Could you check a few things on this model? Use its own coordinates, in mm. Face numbers are marked on the shaded views. Round coordinates to 2 decimals unless told otherwise and drop trailing zeros. Order: outer loops, then holes, each group sorted by start corner. A loop starts at its lowest first (then second) coordinate and runs counter-clockwise, first axis right, second up. Notation, with made-up numbers: (89, 4) - (123, 4) arc R23 cw to (123, 43) - close; hole circle Ø5 at (-28.5, 75.5). An arc over 180 degrees is marked (long way). Use one line per item in the form item = value.
from build123d import *

# Parameters (mm, degrees)
EXTRUDE1_DEPTH          = 6.35
EXTRUDE1_DEPTH_BACK     = 6.35
SKETCH1_R               = 1.4224
SKETCH8_OUTSIDE_W       = 58.916
SKETCH8_OUTSIDE_H       = 59.654
SKETCH8_OUTSIDE_R       = 2.38125
EXTRUDE4_DEPTH          = 14.210632851
EXTRUDE4_DRAFT          = -60
MIRROR1_COPY_1_SKETCH_W = 58.916
MIRROR1_COPY_1_SKETCH_H = 59.654
MIRROR1_COPY_1_SKETCH_R = 2.38125
MIRROR1_COPY_1_DEPTH    = 14.210632851
MIRROR1_COPY_1_DRAFT    = -60


with BuildPart() as part:
    # Sketch1 → Extrude1 (new, two sides: drawn at the far end of the back side and taken through both)
    with BuildSketch(Plane.XY.offset(-EXTRUDE1_DEPTH_BACK)):
        Polygon((0, 2.749630657), (-2.38125, 1.374815329), (-2.38125, -1.374815329), (0, -2.749630657), (2.38125, -1.374815329), (2.38125, 1.374815329), align=None)
        Circle(SKETCH1_R, mode=Mode.SUBTRACT)
    extrude(amount=EXTRUDE1_DEPTH + EXTRUDE1_DEPTH_BACK)

    # Extrude3 cone 1 section (through the dimple's axis) → Extrude3 (revolve, cut)
    with BuildSketch(Plane(origin=(0, 0, -6.35), x_dir=(0, 1, 0), z_dir=(1, 0, 0))):
        Polygon((0, 0), (1.4732, 0), (0, 1.579813584), align=None)
    extrude3 = revolve(axis=Axis((0, 0, -6.35), (0, 0, 1)), mode=Mode.SUBTRACT)


with BuildPart() as extrude4_tool:
    # Sketch8 outside → Extrude4 (with draft: the straight prism first)
    with BuildSketch(Plane(origin=(0, 0, -6.35), x_dir=(-1, 0, 0), z_dir=(0, 0, -1))):
        Rectangle(SKETCH8_OUTSIDE_W, SKETCH8_OUTSIDE_H)
        Circle(SKETCH8_OUTSIDE_R, mode=Mode.SUBTRACT)
    extrude(amount=-EXTRUDE4_DEPTH)
    # Extrude4: the draft: its side faces are tilted about the plane it starts from
    extrude4_sides = [extrude4_tool.faces().sort_by_distance(p)[0] for p in [
        (0, -29.827, 0.755316425),
        (-29.458, 0, 0.755316425),
        (0, 29.827, 0.755316425),
        (29.458, 0, 0.755316425),
        (2.38125, 0, 0.755316425),
    ]]
    draft(extrude4_sides, Plane(origin=(0, 0, -6.35), x_dir=(-1, 0, 0), z_dir=(0, 0, -1)), EXTRUDE4_DRAFT)


with BuildPart() as part_1:
    add(part.part)

    # Extrude4: cut by extrude4_tool
    add(extrude4_tool.part, mode=Mode.SUBTRACT)

    # Mirror1: Extrude3 across plane
    add(extrude3.mirror(Plane.XY), mode=Mode.SUBTRACT)


with BuildPart() as mirror1_copy_1_tool:
    # Mirror1 copy 1 sketch → Mirror1 copy 1 (with draft: the straight prism first)
    with BuildSketch(Plane(origin=(0, 0, 6.35), x_dir=(-1, 0, 0), z_dir=(0, 0, 1))):
        Rectangle(MIRROR1_COPY_1_SKETCH_W, MIRROR1_COPY_1_SKETCH_H)
        Circle(MIRROR1_COPY_1_SKETCH_R, mode=Mode.SUBTRACT)
    extrude(amount=-MIRROR1_COPY_1_DEPTH)
    # Mirror1 copy 1: the draft: its side faces are tilted about the plane it starts from
    mirror1_copy_1_sides = [mirror1_copy_1_tool.faces().sort_by_distance(p)[0] for p in [
        (0, -29.827, -0.755316425),
        (-29.458, 0, -0.755316425),
        (0, 29.827, -0.755316425),
        (29.458, 0, -0.755316425),
        (2.38125, 0, -0.755316425),
    ]]
    draft(mirror1_copy_1_sides, Plane(origin=(0, 0, 6.35), x_dir=(-1, 0, 0), z_dir=(0, 0, 1)), MIRROR1_COPY_1_DRAFT)


with BuildPart() as part_2:
    add(part_1.part)

    # Mirror1 copy 1: cut by mirror1_copy_1_tool
    add(mirror1_copy_1_tool.part, mode=Mode.SUBTRACT)


solid = part_2.part
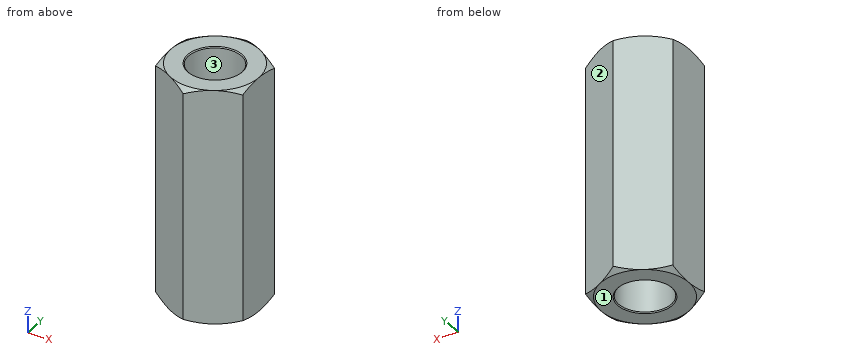
Item 1: Will these pins go through, and if not, where does the flat tip stop? P1, Ø2.5, axis at x = 0, y = 0, coming from the -Z side; P2, Ø2, axis at x = -0.5, z = -2, coming from the +Y side; P3, Ø2, axis at x = 1.5, z = -2.5, coming from the -Y side.
Found:
P1 = through
P2 = 2.75
P3 = -2.46
Item 2: I need wall thicknesses on L1, parallel to X at y = 0, z = -3.5; L2, parallel to X at y = 0.7, z = -4; L3, parallel to X at y = 1.9, z = 6.25. Which ranges of each line are inside material? Lowest first, please.
Found:
L1 = -2.38 to -1.42, 1.42 to 2.38
L2 = -2.38 to -1.24, 1.24 to 2.38
L3 = -1.47 to 1.47
Item 3: Imagine slicing it at A-A on z = -0.75. Please give me the cut outline in (x, y), plus the area to 3 significant figures.
Found:
outline = (-2.38, -1.37) - (0, -2.75) - (2.38, -1.37) - (2.38, 1.37) - (0, 2.75) - (-2.38, 1.37) - close; hole circle Ø2.84 at (0, 0)
area = 13.3 mm2
Item 4: If we mould it in two halves opening along X, with no side actions, what happens to the marked faces 1, 2 and 3? For each: released by +X, released by -X, zero draft, split by the parting line, or undercut.
Found:
face_1 = zero draft
face_2 = released by +X
face_3 = undercut
